Verification items for the finished model (mm, model axes). A direction names the side the tool comes from. Coordinates: 2 decimals unless noted, no trailing zeros. Loops run counter-clockwise (first coordinate to the right, second up) from the corner with the lowest first, then second, coordinate; pieces in that order, holes last.
Q1. Sectioned sample at C-C (y = 58). Enter the section's corners in (x, z), then the cut area to 3 significant figures.
Q2. Sectioned sample at B-B (x = -17). Enter the section's corners in (y, z), then the cut area to 3 significant figures.
Q3. Sectioned sample at D-D (z = 29.5). Enter the section's corners in (x, y), then the cut area to 3 significant figures.
Q4. Material ranges on probe 1 along Y at (x, z) = (-12.5, 98.5); probe 2 along Z at (x, y) = (-103, 10.5); probe 3 along X at (y, z) = (19, 31), recorded low to high.
Q5. Access from +Z, -Z, +X, -X, +Y, -Y to the whole of each face (thin tool, end or side, straight path). Record for faces 5 (the face through (-36.134, 8, 10)), 6 (the face through (-10, 26.559, 77)), 7 (the face through (-73, 40, 20.32)), 8 (the face through (0, 48, 41)), 9 (the face through (-14, 15.24, 14)).
Q6. Go/stop test with flat-tipped pins: P1, Ø5, axis at x = -35.5, y = 35.5, coming from the +Z side; P2, Ø12, axis at x = -11, y = 4.5, coming from the -Z side; P3, Ø4.5, axis at y = 5, z = 14, coming from the +X side; P4, Ø10, axis at y = 35.5, z = 53.5, coming from the -X side. Record where each tip stops, or that it passes through.
Q7. Sectioned sample at A-A (z = 79). Enter the section's corners in (x, y), then the cut area to 3 significant figures.
Q8. Mould release check, pull along Y, two halves, no side actions. Record for faces 1 (the face through (-10, 53.028, 78)), 2 (the face through (-10.018, 40.085, 39.623)), 3 (the face through (-10, 8, 36.134)), 4 (the face through (-60, 0, 10)): +Y half, -Y half, draft (parallel to the pull), parting line (faces both ways), or undercut.
```python
from build123d import *

# Parameters (mm, degrees)
F1_DEPTH = 20.32
F3_DEPTH = 20.32
F4_W     = 36.134478
F4_H     = 36.134478
F5_DEPTH = 15.24


with BuildPart() as f1:
    # F0 (on Right) → F1 (new body)
    with BuildSketch(Plane.YZ):
        with BuildLine():
            Line((0, 102.700152), (0, 0))
            Line((0, 0), (79.587111, 0))
            Line((79.587111, 0), (79.587111, 102.700152))
            Line((79.587111, 102.700152), (53.027965, 102.700152))
            Line((53.027965, 102.700152), (53.027965, 52.854609))
            ThreePointArc((53.027965, 52.854609), (39.793556, 39.620199), (26.559146, 52.854609))
            Line((26.559146, 52.854609), (26.559146, 102.700152))
            Line((26.559146, 102.700152), (0, 102.700152))
        make_face()
    extrude(amount=-F1_DEPTH)

    # F2 (on Top) → F3 (join)
    with BuildSketch(Plane.XY):
        with BuildLine():
            Line((-83.956517, 0), (0, 0))
            Line((0, 0), (0, 79.587111))
            Line((0, 79.587111), (-83.956517, 79.587111))
            ThreePointArc((-83.956517, 79.587111), (-123.750073, 39.793556), (-83.956517, 0))
        make_face()
    extrude(amount=F3_DEPTH)

    # F4 (on Front) → F5 (cut)
    with BuildSketch(Plane.XZ):
        with Locations((-18.067239, 18.067239)):
            Rectangle(F4_W, F4_H)
    extrude(amount=-F5_DEPTH, mode=Mode.SUBTRACT)


solid = f1.part
```
Geometry check:
1. outline: (-119.34, 0) - (0, 0) - (0, 102.7) - (-20.32, 102.7) - (-20.32, 20.32) - (-119.34, 20.32) - close
1. area: 4,100 mm2
2. outline: (0, 36.13) - (15.24, 36.13) - (15.24, 0) - (79.59, 0) - (79.59, 102.7) - (53.03, 102.7) - (53.03, 52.85) arc R13.23 cw to (26.56, 52.85) - (26.56, 102.7) - (0, 102.7) - close
2. area: 6,030 mm2
3. outline: (-20.32, 15.24) - (0, 15.24) - (0, 79.59) - (-20.32, 79.59) - close
3. area: 1,310 mm2
4. probe 1: y = 0 to 26.56, 53.03 to 79.59
4. probe 2: z = 0 to 20.32
4. probe 3: x = -20.32 to 0
5. face 5: +Z, -Z, +X, -Y
5. face 6: +Z, +X, -X
5. face 7: +Z, -X, +Y, -Y
5. face 8: +Z, -Z, +X, +Y, -Y
5. face 9: -Z, +X, -Y
6. P1: stops at z = 20.32
6. P2: stops at z = 36.13
6. P3: stops at x = -36.13
6. P4: passes through
7. outline: (-20.32, 0) - (0, 0) - (0, 26.56) - (-20.32, 26.56) - close; (-20.32, 53.03) - (0, 53.03) - (0, 79.59) - (-20.32, 79.59) - close
7. area: 1,080 mm2
8. face 1: undercut
8. face 2: undercut
8. face 3: draft
8. face 4: -Y half
